Model file for the job. Use its own axes, mm. Face numbers are marked on the shaded views. A direction names the side the tool comes from. Round coordinates to 2 decimals unless told otherwise and drop trailing zeros. Loops run counter-clockwise (first coordinate to the right, second up) from the corner with the lowest first, then second, coordinate; pieces in that order, holes last. Notation, with made-up numbers: (65, -23.5) - (94, -23.5) arc R24 ccw to (94, 9.5) - close; hole circle Ø10 at (-13.5, 36). An arc over 180 degrees is marked (long way). Answer as a JSON object with one key per item and string values.
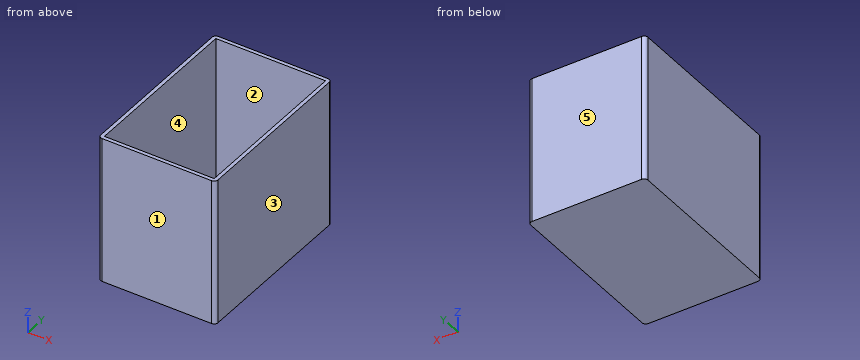
from build123d import *

# Parameters (mm, degrees)
F1_DEPTH = 127
F2_T     = 3.175


# Not quite as in the source:
# - a shell that OpenCascade refuses in one call is made with other operations: the cavity is built on its own and cut out


with BuildPart() as f1:
    # F0 (on Top) → F1 (new body)
    with BuildSketch(Plane.XY):
        with BuildLine():
            ThreePointArc((50.8, 73.025), (49.8700640303, 75.2700640303), (47.625, 76.2))
            Line((47.625, 76.2), (-47.625, 76.2))
            ThreePointArc((-47.625, 76.2), (-49.8700640303, 75.2700640303), (-50.8, 73.025))
            Line((-50.8, 73.025), (-50.8, -73.025))
            ThreePointArc((-50.8, -73.025), (-49.8700640303, -75.2700640303), (-47.625, -76.2))
            Line((-47.625, -76.2), (47.625, -76.2))
            ThreePointArc((47.625, -76.2), (49.8700640303, -75.2700640303), (50.8, -73.025))
            Line((50.8, -73.025), (50.8, 73.025))
        make_face()
    extrude(amount=F1_DEPTH)

    # F2: shell of thickness 3.175, made by hand


with BuildPart() as f2_core1:
    # F2_t2: copy of F1
    add(f1.part)

    # the walls: a layer under each face that stays
    f2_faces = [f2_core1.faces().sort_by_distance(p)[0] for p in [
        (0, 76.2, 63.5),
        (-50.8, 0, 63.5),
        (0, -76.2, 63.5),
        (50.8, 0, 63.5),
        (0, 0, 0),
    ]]
    thicken(f2_faces, amount=-F2_T, mode=Mode.SUBTRACT)


with BuildPart() as f1_1:
    add(f1.part)

    # what is left inside the walls is the cavity
    f2_cavity = [f2_core1.part.solids().sort_by_distance(p)[0] for p in [
        (47.59325, 0, 85.725),
    ]]
    add(f2_cavity, mode=Mode.SUBTRACT)


solid = f1_1.part
1) Slice it at B-B on z = 88. List the corners of the cut face in (x, y) (3 decimals), then the cut area to 3 significant figures.
Values follow:
{"outline": "(-50.8, -73.025) arc R3.175 ccw to (-47.625, -76.2) - (47.625, -76.2) arc R3.175 ccw to (50.8, -73.025) - (50.8, 73.025) arc R3.175 ccw to (47.625, 76.2) - (-47.625, 76.2) arc R3.175 ccw to (-50.8, 73.025) - close; hole (-47.625, -73.025) - (47.625, -73.025) - (47.625, 73.025) - (-47.625, 73.025) - close", "area": "1,560 mm²"}
2) Two-plate mould, pull along X, no slides. Class the marked faces 1, 2 and 3: pulls with the +X half, pulls with the -X half, needs draft (parallel to the pull), parting line crosses it, or undercut.
Values follow:
{"face 1": "needs draft", "face 2": "undercut", "face 3": "pulls with the +X half"}
3) Drop a flat-ended pin along its axis: P1, Ø6, axis at x = -22.5, y = 1.5, coming from the +Z side (3 decimals). Give the stop position or say it passes through.
Values follow:
{"P1": "z = 3.175"}
4) Probe probe 1 along X at (y, z) = (54, 27) (3 decimals); probe 2 along Y at (x, z) = (-16.5, 67.5) (3 decimals); probe 3 along Z at (x, y) = (-20.5, 1) (3 decimals). List the from-to ranges inside material, lowest first.
Values follow:
{"probe 1": "-50.8 to -47.625, 47.625 to 50.8", "probe 2": "-76.2 to -73.025, 73.025 to 76.2", "probe 3": "0 to 3.175"}
5) Slice it at A-A on x = -15. List the corners of the cut face in (y, z) (3 decimals).
Values follow:
{"outline": "(-76.2, 0) - (76.2, 0) - (76.2, 127) - (73.025, 127) - (73.025, 3.175) - (-73.025, 3.175) - (-73.025, 127) - (-76.2, 127) - close"}
6) Tool access for the marked faces 4 and 5: list every direction of +Z, -Z, +X, -X, +Y, -Y with a clear straight run to the whole face (end or side of a thin tool).
Values follow:
{"face 4": "+Z", "face 5": "+Z, -Z, +X, -X, +Y"}
7) Slice it at C-C on y = -43.5. List the corners of the cut face in (x, z) (3 decimals), then the cut area to 3 significant figures.
Values follow:
{"outline": "(-50.8, 0) - (50.8, 0) - (50.8, 127) - (47.625, 127) - (47.625, 3.175) - (-47.625, 3.175) - (-47.625, 127) - (-50.8, 127) - close", "area": "1,110 mm²"}
